```python
from build123d import *

# Parameters (mm, degrees)
SKETCH1_W           = 250
SKETCH1_H           = 150
BOSS_EXTRUDE1_DEPTH = 40
FILLET1_START       = -75
FILLET1_DEPTH       = 150
FILLET1_START_2     = -126
FILLET1_2_DEPTH     = 252


with BuildPart() as part:
    # Sketch1 → Boss-Extrude1 (new body)
    with BuildSketch(Plane(origin=(0, 0, 0), x_dir=(1, 0, 0), z_dir=(0, 1, 0))):
        Rectangle(SKETCH1_W, SKETCH1_H)
    extrude(amount=BOSS_EXTRUDE1_DEPTH)

    # Fillet1: read off the stored shape, not the designer's step
    # Fillet1 outline → Fillet1 (cut)
    with BuildSketch(Plane.XY.offset(FILLET1_START)):
        with BuildLine():
            Line((-125, 40), (-125, 20))
            ThreePointArc((-125, 20), (-119.142135624, 34.142135624), (-105, 40))
            Line((-105, 40), (-125, 40))
        make_face()
        with BuildLine():
            Line((125, 40), (105, 40))
            ThreePointArc((105, 40), (119.142135624, 34.142135624), (125, 20))
            Line((125, 20), (125, 40))
        make_face()
    extrude(amount=FILLET1_DEPTH, mode=Mode.SUBTRACT)

    # Fillet1 2 outline → Fillet1 2 (cut)
    with BuildSketch(Plane.YZ.offset(FILLET1_START_2)):
        with BuildLine():
            Line((40, 75), (20, 75))
            ThreePointArc((20, 75), (34.142135624, 69.142135624), (40, 55))
            Line((40, 55), (40, 75))
        make_face()
        with BuildLine():
            Line((40, -75), (40, -55))
            ThreePointArc((40, -55), (34.142135624, -69.142135624), (20, -75))
            Line((20, -75), (40, -75))
        make_face()
    extrude(amount=FILLET1_2_DEPTH, mode=Mode.SUBTRACT)


solid = part.part
```
Geometry: final body of the model. Coordinates: model frame, mm. Coordinates: 2 decimals unless noted, no trailing zeros. Loops run counter-clockwise (first coordinate to the right, second up) from the corner with the lowest first, then second, coordinate; pieces in that order, holes last. Notation, with made-up numbers: (15, 46.25) -> (32, 46.25) arc R22 ccw to (32, 56.25) -> close; hole circle Ø6 at (30, 27.25). An arc over 180 degrees is marked (long way). Use a Markdown table: item, result. Add a question column.
(1) Section query C-C, the plane z = 0.5. Return loops of the section in (x, y).
(2) Section query A-A, the plane x = -67. Return loops of the section in (y, z), plus the area to 3 significant figures.
(3) Pin query (flat end, axial travel): pin 1 Ø3 at (y, z) = (35, 16.5) entering from +X; pin 2 Ø2 at (y, z) = (24, -58.5) entering from -X; pin 3 Ø1 at (y, z) = (32, 13) entering from +X. Return the tip coordinate at first contact, or that it passes through.
(4) Line query: line 1 along Z through (x, y) = (78.5, 37); line 2 along X through (y, z) = (33.5, -20); line 3 along X through (y, z) = (27, 47.5) (3 decimals). Output: solid intervals per line, ascending.
(5) Section query B-B, the plane y = 36. Return loops of the section in (x, z).
Answer:
| question | item | result |
|---|---|---|
| 1 | outline | (-125, 0) -> (125, 0) -> (125, 20) arc R20 ccw to (105, 40) -> (-105, 40) arc R20 ccw to (-125, 20) -> close |
| 2 | outline | (0, -75) -> (20, -75) arc R20 ccw to (40, -55) -> (40, 55) arc R20 ccw to (20, 75) -> (0, 75) -> close |
| 2 | area | 5,830 mm^2 |
| 3 | pin 1 | stops at x = 119.76 |
| 3 | pin 2 | stops at x = -124.77 |
| 3 | pin 3 | stops at x = 121.36 |
| 4 | line 1 | z = -65.54 to 65.54 |
| 4 | line 2 | x = -119.76 to 119.76 |
| 4 | line 3 | x = -123.735 to 123.735 |
| 5 | outline | (-117, -67) -> (117, -67) -> (117, 67) -> (-117, 67) -> close |
